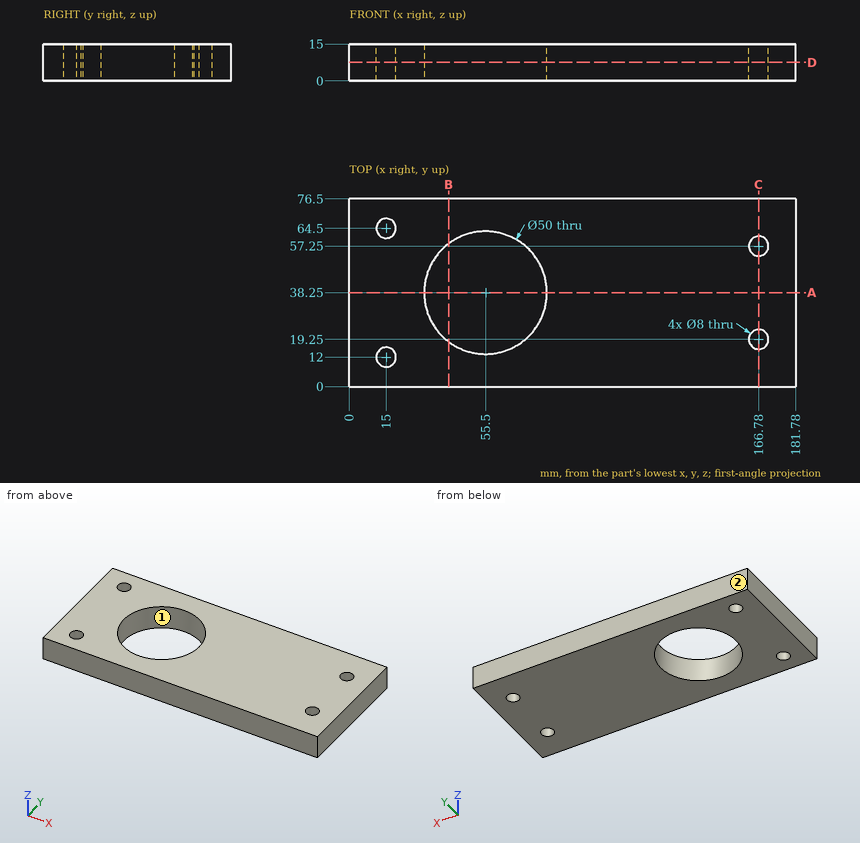
Design review of the part shown in the three views and the two pictorial views. Dimensions are in mm from the part's minimum x, y and z. Round coordinates to 2 decimals unless told otherwise and drop trailing zeros. Write each loop counter-clockwise with the first axis right and the second up, starting at its lowest first coordinate (ties: lowest second). Pieces come first, ordered by that corner, then holes. Notation, with made-up numbers: (50, 43) -> (90, 43) arc R34 cw to (90, 73) -> close; hole circle Ø8 at (-23.5, 84). An arc over 180 degrees is marked (long way). Answer as a JSON object with one key per item and string values.
1. We need section C-C on x = 166.78. State the section outline as (y, z) points, and give its area (4 significant figures).
Results found:
{"outline": "(0, 0) -> (15.25, 0) -> (15.25, 15) -> (0, 15) -> close; (23.25, 0) -> (53.25, 0) -> (53.25, 15) -> (23.25, 15) -> close; (61.25, 0) -> (76.5, 0) -> (76.5, 15) -> (61.25, 15) -> close", "area": "907.5 mm^2"}
2. Clearance check with a flat-ended pin moving along its axis: pin 1 (5 mm diameter, centred on x = 166.78, y = 19.25, fed in from -Z). State where the tip first meets the part, or that it passes through.
Results found:
{"pin 1": "passes through"}
3. The part is to be moulded in two halves that separate along X. For the marked faces 1 and 2, say which applies: pulls with the +X half, pulls with the -X half, needs draft (parallel to the pull), parting line crosses it, or undercut.
Results found:
{"face 1": "undercut", "face 2": "needs draft"}
4. We need section A-A on y = 38.25. State the section outline as (x, z) points, and give its area (3 significant figures).
Results found:
{"outline": "(0, 0) -> (30.5, 0) -> (30.5, 15) -> (0, 15) -> close; (80.5, 0) -> (181.78, 0) -> (181.78, 15) -> (80.5, 15) -> close", "area": "1,980 mm^2"}
5. We need section D-D on z = 7.5. State the section outline as (x, y) points.
Results found:
{"outline": "(0, 0) -> (181.78, 0) -> (181.78, 76.5) -> (0, 76.5) -> close; hole circle Ø8 at (15, 12); hole circle Ø8 at (15, 64.5); hole circle Ø50 at (55.5, 38.25); hole circle Ø8 at (166.78, 19.25); hole circle Ø8 at (166.78, 57.25)"}
6. To check wall thickness, follow line 1 along Y through (x, z) = (15, 9.25); line 2 along Y through (x, z) = (166.78, 9); line 3 along X through (y, z) = (12, 10.25). State the ranges of each line that lie inside material, in increasing order.
Results found:
{"line 1": "y = 0 to 8, 16 to 60.5, 68.5 to 76.5", "line 2": "y = 0 to 15.25, 23.25 to 53.25, 61.25 to 76.5", "line 3": "x = 0 to 11, 19 to 181.78"}
7. We need section B-B on x = 40.5. State the section outline as (y, z) points, and give its area (4 significant figures).
Results found:
{"outline": "(0, 0) -> (18.25, 0) -> (18.25, 15) -> (0, 15) -> close; (58.25, 0) -> (76.5, 0) -> (76.5, 15) -> (58.25, 15) -> close", "area": "547.5 mm^2"}
